from build123d import *

# Parameters (mm, degrees)
BOSS_EXTRUDE1_DEPTH       = 14
SKETCH2_W                 = 45
SKETCH2_H                 = 10.2
CUT_EXTRUDE1_DEPTH        = 15
F_4_CLEARANCE_HOLE1_D     = 3.3
F_4_CLEARANCE_HOLE1_DEPTH = 14
F_4_CLEARANCE_HOLE2_D     = 3.3
F_4_CLEARANCE_HOLE2_DEPTH = 19.899999999
F_8_CLEARANCE_HOLE1_D     = 4.5
F_8_CLEARANCE_HOLE1_DEPTH = 14
CHAMFER1_SIZE             = 2.45
FILLET1_R                 = 10


with BuildPart() as part:
    # Sketch1 → Boss-Extrude1 (new body)
    with BuildSketch(Plane.XY.offset(14)):
        with BuildLine():
            Line((125, 0), (0, 0))
            Line((0, 0), (0, -50))
            Line((0, -50), (125, -50))
            ThreePointArc((125, -50), (150, -25), (125, 0))
        make_face()
    extrude(amount=-BOSS_EXTRUDE1_DEPTH)

    # Sketch2 → Cut-Extrude1 (cut, through all)
    with BuildSketch(Plane(origin=(0, 0, 0), x_dir=(-1, 0, 0), z_dir=(0, 0, -1))):
        with Locations((-22.5, -24.999999999)):
            Rectangle(SKETCH2_W, SKETCH2_H)
    extrude(amount=-CUT_EXTRUDE1_DEPTH, mode=Mode.SUBTRACT)

    # Sketch3 → Cut-Revolve1 (revolve, cut)
    with BuildSketch(Plane(origin=(0, -24.999999999, 0), x_dir=(1, 0, 0), z_dir=(0, 1, 0))):
        Polygon((127.3, 0), (123.999999995, 0), (123.999999995, -14), (144, -14), (144, -3), (139.5, -3), (139.5, -2), (127.3, -2), align=None)
    revolve(axis=Axis((123.999999995, -24.999999999, 0), (0, 0, 1)), mode=Mode.SUBTRACT)

    # #4 Clearance Hole1
    with Locations(Plane(origin=(0, 0, 0), x_dir=(-1, 0, 0), z_dir=(0, 0, -1))):
        with Locations((-70, -8)):
            Hole(F_4_CLEARANCE_HOLE1_D / 2, depth=F_4_CLEARANCE_HOLE1_DEPTH)

    # #4 Clearance Hole2
    with Locations(Plane(origin=(0, 0, 0), x_dir=(1, 0, 0), z_dir=(0, 1, 0))):
        with Locations((24.5, -7), (41.7, -7)):
            Hole(F_4_CLEARANCE_HOLE2_D / 2, depth=F_4_CLEARANCE_HOLE2_DEPTH)

    # #8 Clearance Hole1
    with Locations(Plane(origin=(0, 0, 0), x_dir=(-1, 0, 0), z_dir=(0, 0, -1))):
        with Locations((-15, -8), (-15, -42), (-35, -42), (-35, -8), (-55, -8), (-55, -42)):
            Hole(F_8_CLEARANCE_HOLE1_D / 2, depth=F_8_CLEARANCE_HOLE1_DEPTH)

    # Chamfer1
    chamfer1_edges = [part.edges().sort_by_distance(p)[0] for p in [
        (52.75, -42, 0),
        (52.75, -8, 0),
        (32.75, -8, 0),
        (32.75, -42, 0),
        (12.75, -42, 0),
        (12.75, -8, 0),
    ]]
    chamfer(chamfer1_edges, length=CHAMFER1_SIZE)

    # Fillet1
    fillet1_edges = [part.edges().sort_by_distance(p)[0] for p in [
        (0, -9.95, 0),
        (0, -40.05, 0),
    ]]
    fillet(fillet1_edges, radius=FILLET1_R)


solid = part.part
CAD build for the part. Positions are in the model's coordinates, mm. A direction names the side the tool comes from. Coordinates: 2 decimals unless noted, no trailing zeros. Write each loop counter-clockwise with the first axis right and the second up, starting at its lowest first coordinate (ties: lowest second). Pieces come first, ordered by that corner, then holes. Notation, with made-up numbers: M 4.25,2.5 L 40.25,2.5 A26 ccw 40.25,39.5 Z; hole C 26.25,19.5 d11. An arc over 180 degrees is marked long. Return JSON: item names as keys, results as strings.
Item 1: Probe line 1 (Y direction, x = 15, z = 5); line 2 (Y direction, x = 124, z = 0.7); line 3 (Y direction, x = 11, z = 1.5). List the from-to ranges inside material, lowest first. Write a range as from..to.
Findings below:
{"line 1": "y = -50..-44.25, -39.75..-30.1, -19.9..-10.25, -5.75..0", "line 2": "y = -50..-28.3, -21.7..0", "line 3": "y = -50..-30.1, -19.9..0"}
Item 2: Slice it at A-A, the plane y = -25. Write the cut outline in (x, z).
Findings below:
{"outline": "M 45,0 L 120.7,0 L 120.7,2 L 108.5,2 L 108.5,3 L 104,3 L 104,14 L 45,14 Z; M 127.3,0 L 150,0 L 150,14 L 144,14 L 144,3 L 139.5,3 L 139.5,2 L 127.3,2 Z"}
Item 3: Slice it at B-B, the plane x = 41.7. Write the cut outline in (y, z).
Findings below:
{"outline": "M -50,0 L -30.1,0 L -30.1,14 L -50,14 Z; M -19.9,0 L 0,0 L 0,5.35 L -19.9,5.35 Z; M -19.9,8.65 L 0,8.65 L 0,14 L -19.9,14 Z"}
Item 4: Drop flat-ended pins along their axis: pin 1 Ø3 at (x, y) = (70, -8) entering from +Z; pin 2 Ø6 at (y, z) = (-29.5, 4.5) entering from -X; pin 3 Ø15.5 at (x, y) = (130.5, -17.5) entering from +Z; pin 4 Ø24 at (x, y) = (124, -25) entering from +Z. Give the stop position or say it passes through.
Findings below:
{"pin 1": "passes through", "pin 2": "stops at x = 0.33", "pin 3": "stops at z = 3", "pin 4": "stops at z = 2"}
Item 5: Slice it at C-C, the plane z = 12. State how many separate pieces and enclosed holes the cut face has, and give its area (3 significant figures).
Findings below:
{"separate pieces": "1", "enclosed holes": "8", "area": "5,410 mm2"}
Item 6: Slice it at D-D, the plane x = 70. Write the cut outline in (y, z).
Findings below:
{"outline": "M -50,0 L -9.65,0 L -9.65,14 L -50,14 Z; M -6.35,0 L 0,0 L 0,14 L -6.35,14 Z"}
Item 7: Which spindle directions (+Z, -Z, +X, -X, +Y, -Y) get a long thin tool onto all of the face, cutting with end or side? Do faces 4 (the flat face through (23, -19.9, 8)), 5 (the cylindrical face through (143.076, -18.993, 8.423)), 6 (the flat face through (0, -40, 12)). Say none if no direction does.
Findings below:
{"face 4": "+Z, -Z, -X", "face 5": "+Z", "face 6": "+Z, -Z, -X, +Y, -Y"}
Item 8: Two-plate mould, pull along Y, no slides. Class faces 1 (the flat face through (62, -50, 7)), 2 (the flat face through (79, -25, 0)), 3 (the conical face through (12.6, -7.9, 2.3)): +Y half, -Y half, draft (parallel to the pull), parting line (faces both ways), or undercut.
Findings below:
{"face 1": "-Y half", "face 2": "draft", "face 3": "undercut"}
